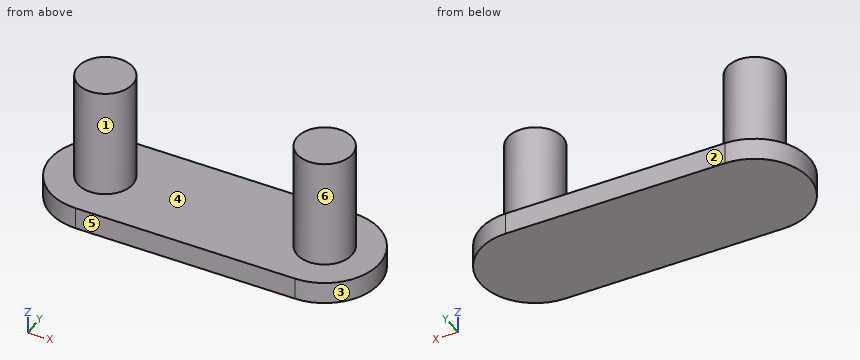
Solid Edge part; units mm, degrees
sketch "Sketch1" plane through (0, 0, 0) normal (0, 0, 1) x (1, 0, 0)
  line L0 (-10, 5) -> (10, 5)
  line L1 (-10, -5) -> (10, -5)
  arc A0 (-10, -5) -> (-10, 5) centre (-10, 0) cw
  arc A1 (10, 5) -> (10, -5) centre (10, 0) cw
extrude "Protrusion1" add sketch "Sketch1" against normal blind 2
sketch "Sketch2" plane through (0, 0, 0) normal (0, 0, 1) x (1, 0, 0)
  circle A0 centre (-10, 0) radius 2.5
  circle A1 centre (10, 0) radius 2.5
extrude "ExtrudedProtrusion_2" add sketch "Sketch2" along normal blind 10
Geometry: final body of the model. Coordinates: model frame, mm. Face numbers are marked on the shaded views. A direction names the side the tool comes from. Round coordinates to 2 decimals unless told otherwise and drop trailing zeros. Write each loop counter-clockwise with the first axis right and the second up, starting at its lowest first coordinate (ties: lowest second). Pieces come first, ordered by that corner, then holes. Notation, with made-up numbers: M 76,16 L 132,16 A11 cw 132,36 Z; hole C 31,-30 d3. An arc over 180 degrees is marked long. Answer in a Markdown table with one row per item. Add a question column.
(1) Cut plane C-C, the plane x = 0. Return the cut outline in (y, z), then the cut area to 3 significant figures.
(2) Contact query for a flat-ended pin moving along its axis: pin 1 (4 mm diameter, centred on x = 0.5, y = 1.5, fed in from +Z). Output: stop coordinate, or through.
(3) Draft query along X for the marked faces 1, 2, 3 and 4. Return one class per face: pulls with the +X half, pulls with the -X half, needs draft (parallel to the pull), parting line crosses it, or undercut.
(4) Reachability of the marked faces 5 and 6 from +Z, -Z, +X, -X, +Y, -Y: full face, straight path, thin tool, end or side. Return the list, or none.
(5) Ray query, L1, parallel to Z at x = -2, y = 0.75; L2, parallel to X at y = 2, z = 5.25; L3, parallel to X at y = 0.75, z = 3. Return the intervals inside material, ascending.
(6) Cut plane A-A, the plane y = 0. Return the cut outline in (x, z).
(7) Cut plane D-D, the plane y = 4. Return the cut outline in (x, z).
(8) Cut plane B-B, the plane z = 1.75. Return the cut outline in (x, y), then the cut area to 3 significant figures.
Established:
| question | item | result |
|---|---|---|
| 1 | outline | M -5,-2 L 5,-2 L 5,0 L -5,0 Z |
| 1 | area | 20.0 mm² |
| 2 | pin 1 | z = 0 |
| 3 | face 1 | undercut |
| 3 | face 2 | needs draft |
| 3 | face 3 | pulls with the +X half |
| 3 | face 4 | undercut |
| 4 | face 5 | +Z, -Z, +X, -X, -Y |
| 4 | face 6 | +Z |
| 5 | L1 | -2 to 0 |
| 5 | L2 | -11.5 to -8.5, 8.5 to 11.5 |
| 5 | L3 | -12.38 to -7.62, 7.62 to 12.38 |
| 6 | outline | M -15,-2 L 15,-2 L 15,0 L 12.5,0 L 12.5,10 L 7.5,10 L 7.5,0 L -7.5,0 L -7.5,10 L -12.5,10 L -12.5,0 L -15,0 Z |
| 7 | outline | M -13,-2 L 13,-2 L 13,0 L -13,0 Z |
| 8 | outline | C -10,0 d5; C 10,0 d5 |
| 8 | area | 39.3 mm² |
